Input: dimensioned drawing with shaded views. Units: mm. Origin: part minimum x, y, z. A direction names the side the tool comes from. Round coordinates to 2 decimals unless told otherwise and drop trailing zeros. Loops run counter-clockwise (first coordinate to the right, second up) from the corner with the lowest first, then second, coordinate; pieces in that order, holes last.
1) Ray query, line 1 along Y through (x, z) = (21.2, 26); line 2 along X through (y, z) = (38, 36.5); line 3 along Z through (x, y) = (14.75, 26). Return the intervals inside material, ascending.
2) Access query for the marked faces 1 and 2. Directions: +Z, -Z, +X, -X, +Y, -Y. A direction counts if a zero-diameter tool reaches every point of the face in a straight line with its end or side. Return the directions, or none.
3) First-contact query: pin 1 (1.8 mm diameter, centred on y = 45.5, z = 26, fed in from -X); pin 2 (6 mm diameter, centred on x = 14.5, z = 32.5, fed in from +Y); pin 3 (1 mm diameter, centred on x = 11.5, z = 23.5, fed in from -Y); pin 4 (10 mm diameter, centred on x = 14.5, y = 35.5, fed in from -Z). Flat tips, straight axial feed; report the tip coordinate or a pass-through.
4) Section A-A, the plane y = 26. Return loops of the section in (x, z).
5) Draft query along X for the marked faces 3, 4 and 5. Return one class per face: pulls with the +X half, pulls with the -X half, needs draft (parallel to the pull), parting line crosses it, or undercut.
6) Section C-C, the plane y = 45.5. Return loops of the section in (x, z).
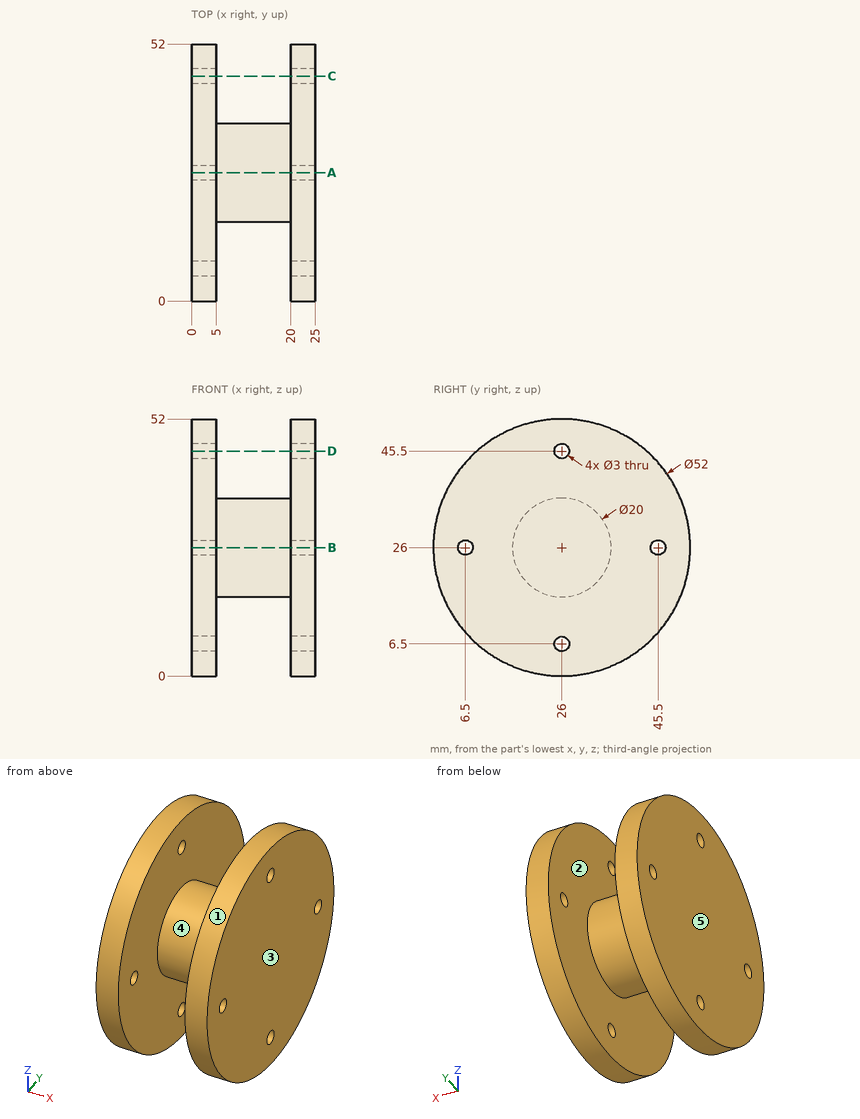
Final values:
1. line 1: y = 0 to 5, 8 to 44, 47 to 52
1. line 2: x = 0 to 5, 20 to 25
1. line 3: z = 16 to 36
2. face 1: +X, -X
2. face 2: none
3. pin 1: passes through
3. pin 2: stops at y = 35.37
3. pin 3: stops at y = 16.2
3. pin 4: stops at z = 17.07
4. outline: (0, 0) - (5, 0) - (5, 5) - (0, 5) - close; (0, 8) - (5, 8) - (5, 16) - (20, 16) - (20, 8) - (25, 8) - (25, 44) - (20, 44) - (20, 36) - (5, 36) - (5, 44) - (0, 44) - close; (0, 47) - (5, 47) - (5, 52) - (0, 52) - close; (20, 0) - (25, 0) - (25, 5) - (20, 5) - close; (20, 47) - (25, 47) - (25, 52) - (20, 52) - close
5. face 3: pulls with the +X half
5. face 4: undercut
5. face 5: pulls with the -X half
6. outline: (0, 8.8) - (5, 8.8) - (5, 24.5) - (0, 24.5) - close; (0, 27.5) - (5, 27.5) - (5, 43.2) - (0, 43.2) - close; (20, 8.8) - (25, 8.8) - (25, 24.5) - (20, 24.5) - close; (20, 27.5) - (25, 27.5) - (25, 43.2) - (20, 43.2) - close
